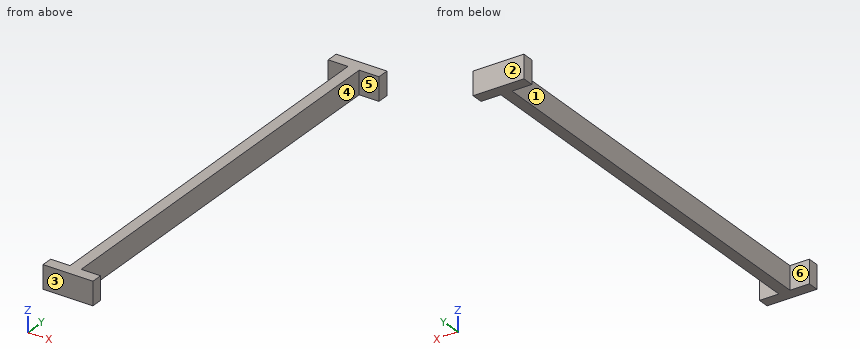
from build123d import *

# Parameters (mm, degrees)
SKETCH1_W           = 4.8
SKETCH1_H           = 2.351445648
SKETCH1_W_2         = 21.4
SKETCH1_H_2         = 4.8
BOSS_EXTRUDE1_DEPTH = 10
SKETCH2_W           = 4.8
SKETCH2_H           = 10
BOSS_EXTRUDE2_DEPTH = 177.5
SKETCH4_W           = 10
SKETCH4_H           = 5
BOSS_EXTRUDE6_DEPTH = 8.5
SKETCH8_W           = 10
SKETCH8_H           = 5
BOSS_EXTRUDE7_DEPTH = 8.5


with BuildPart() as part:
    # Sketch1 → Boss-Extrude1 (new body)
    with BuildSketch(Plane.XY):
        with Locations((-0.408910891, -0.704145163)):
            Rectangle(SKETCH1_W, SKETCH1_H)
        with Locations((-0.408910891, -4.279867987)):
            Rectangle(SKETCH1_W_2, SKETCH1_H_2)
    extrude(amount=BOSS_EXTRUDE1_DEPTH)

    # Sketch2 → Boss-Extrude2 (add)
    with BuildSketch(Plane(origin=(0, 0.471577661, 0), x_dir=(1, 0, 0), z_dir=(0, 1, 0))):
        with Locations((-0.408910891, -5)):
            Rectangle(SKETCH2_W, SKETCH2_H)
    extrude(amount=BOSS_EXTRUDE2_DEPTH)

    # Sketch4 → Boss-Extrude6 (add)
    with BuildSketch(Plane(origin=(1.991089109, 0, 0), x_dir=(0, 0, -1), z_dir=(1, 0, 0))):
        with Locations((-5, 175.471577661)):
            Rectangle(SKETCH4_W, SKETCH4_H)
    extrude(amount=BOSS_EXTRUDE6_DEPTH)

    # Sketch8 → Boss-Extrude7 (add)
    with BuildSketch(Plane.ZY.offset(2.808910891)):
        with Locations((5, 175.471577661)):
            Rectangle(SKETCH8_W, SKETCH8_H)
    extrude(amount=BOSS_EXTRUDE7_DEPTH)


solid = part.part
Work out the finished part from the listing and answer in its coordinate system (mm). Face numbers are marked on the shaded views. A direction names the side the tool comes from. Coordinates: 2 decimals unless noted, no trailing zeros. Write each loop counter-clockwise with the first axis right and the second up, starting at its lowest first coordinate (ties: lowest second). Pieces come first, ordered by that corner, then holes. Notation, with made-up numbers: M 10,15 L 60,15 A29 ccw 60,49 Z; hole C 5,73 d6. An arc over 180 degrees is marked long. Write item = value, one per line.
1. The part is cut by section A-A (x = -7.5). Determine the outline of the cut face in (y, z).
Solution:
outline = M -6.68,0 L -1.88,0 L -1.88,10 L -6.68,10 Z; M 172.97,0 L 177.97,0 L 177.97,10 L 172.97,10 Z
2. The part is cut by section C-C (y = 50.5). Determine the outline of the cut face in (x, z), then the cut area to 3 significant figures.
Solution:
outline = M -2.81,0 L 1.99,0 L 1.99,10 L -2.81,10 Z
area = 48.0 mm2
3. The part is cut by section B-B (z = 2). Determine the outline of the cut face in (x, y), then the cut area to 3 significant figures.
Solution:
outline = M -11.31,172.97 L -2.81,172.97 L -2.81,-1.88 L -11.11,-1.88 L -11.11,-6.68 L 10.29,-6.68 L 10.29,-1.88 L 1.99,-1.88 L 1.99,172.97 L 10.49,172.97 L 10.49,177.97 L -11.31,177.97 Z
area = 1,050 mm2
4. Straight lines are drawn through the part: line 1 (Y direction, x = -6, z = 0.5); line 2 (X direction, y = 121, z = 2.25). For each, find the intervals that lie inside material, in ascending order. Write a range as from..to.
Solution:
line_1 = -6.68..-1.88, 172.97..177.97
line_2 = -2.81..1.99
5. Flat-ended cylindrical pins translate along their axes: pin 1 (4 mm diameter, centred on y = 152.5, z = 3, fed in from +X); pin 2 (2.5 mm diameter, centred on y = -3.5, z = 7, fed in from -X); pin 3 (3 mm diameter, centred on y = 23.5, z = 5, fed in from -X). Find the tip coordinate at first contact, or state that the pin passes through.
Solution:
pin_1 = 1.99
pin_2 = -11.11
pin_3 = -2.81
6. For the marked faces 5 and 6, determine the directions among +Z, -Z, +X, -X, +Y, -Y from which every point of the face is accessible in a straight line to the end or side of a thin tool.
Solution:
face_5 = +Z, -Z, +X
face_6 = +Z, -Z, -X
7. Determine the mould class of the marked faces 1, 2, 3 and 4 for opening direction Y: released by +Y, released by -Y, zero draft, split by the parting line, or undercut.
Solution:
face_1 = undercut
face_2 = released by +Y
face_3 = released by -Y
face_4 = undercut
